Design review of the part built by this model. Coordinates are the model's own, in mm. Face numbers are marked on the shaded views. Round coordinates to 2 decimals unless told otherwise and drop trailing zeros. Order: outer loops, then holes, each group sorted by start corner. A loop starts at its lowest first (then second) coordinate and runs counter-clockwise, first axis right, second up.
from build123d import *

# Parameters (mm, degrees)
SKETCH_1_W          = 420
SKETCH_1_H          = 60
EXTRUDE_1_DEPTH     = 8
SKETCH_2_R          = 30
EXTRUDE_2_DEPTH     = 8
SKETCH_3_W          = 420
SKETCH_3_H          = 8
EXTRUDE_3_DEPTH     = 8
SKETCH_4_R          = 10
CUT_EXTRUDE_1_DEPTH = 481
SKETCH_5_R          = 8
CUT_EXTRUDE_2_DEPTH = 481
CUT_EXTRUDE_3_DEPTH = 455.264240283


with BuildPart() as part:
    # 草图1 → 凸台-拉伸1 (new body)
    with BuildSketch(Plane.XY):
        with Locations((210, 30)):
            Rectangle(SKETCH_1_W, SKETCH_1_H)
    extrude(amount=EXTRUDE_1_DEPTH)

    # 草图2 → 凸台-拉伸2 (add)
    with BuildSketch(Plane.XY):
        with Locations((0, 30)):
            Circle(SKETCH_2_R)
        with Locations((420, 30)):
            Circle(SKETCH_2_R)
    extrude(amount=EXTRUDE_2_DEPTH)

    # 草图3 → 凸台-拉伸3 (add)
    with BuildSketch(Plane.XY.offset(8)):
        with Locations((210, 4)):
            Rectangle(SKETCH_3_W, SKETCH_3_H)
        with Locations((210, 56)):
            Rectangle(SKETCH_3_W, SKETCH_3_H)
    extrude(amount=EXTRUDE_3_DEPTH)

    # 草图4 → 切除-拉伸1 (cut, symmetric)
    with BuildSketch(Plane.XY.offset(8)):
        with Locations((0, 30)):
            Circle(SKETCH_4_R)
    extrude(amount=CUT_EXTRUDE_1_DEPTH, both=True, mode=Mode.SUBTRACT)

    # 草图5 → 切除-拉伸2 (cut, symmetric)
    with BuildSketch(Plane.XY.offset(8)):
        with Locations((420, 30)):
            Circle(SKETCH_5_R)
    extrude(amount=CUT_EXTRUDE_2_DEPTH, both=True, mode=Mode.SUBTRACT)

    # 草图6 → 切除-拉伸3 (cut, through all)
    with BuildSketch(Plane.XY):
        with BuildLine():
            Line((28, 10), (72, 10))
            ThreePointArc((72, 10), (75.577708764, 12.211145618), (75.2, 16.4))
            Line((75.2, 16.4), (53.2, 45.733333333))
            ThreePointArc((53.2, 45.733333333), (50, 47.333333333), (46.8, 45.733333333))
            Line((46.8, 45.733333333), (24.8, 16.4))
            ThreePointArc((24.8, 16.4), (24.422291236, 12.211145618), (28, 10))
        make_face()
        with BuildLine():
            Line((108, 10), (152, 10))
            ThreePointArc((152, 10), (155.577708764, 12.211145618), (155.2, 16.4))
            Line((155.2, 16.4), (133.2, 45.733333333))
            ThreePointArc((133.2, 45.733333333), (130, 47.333333333), (126.8, 45.733333333))
            Line((126.8, 45.733333333), (104.8, 16.4))
            ThreePointArc((104.8, 16.4), (104.422291236, 12.211145618), (108, 10))
        make_face()
        with BuildLine():
            Line((188, 10), (232, 10))
            ThreePointArc((232, 10), (235.577708764, 12.211145618), (235.2, 16.4))
            Line((235.2, 16.4), (213.2, 45.733333333))
            ThreePointArc((213.2, 45.733333333), (210, 47.333333333), (206.8, 45.733333333))
            Line((206.8, 45.733333333), (184.8, 16.4))
            ThreePointArc((184.8, 16.4), (184.422291236, 12.211145618), (188, 10))
        make_face()
        with BuildLine():
            Line((268, 10), (312, 10))
            ThreePointArc((312, 10), (315.577708764, 12.211145618), (315.2, 16.4))
            Line((315.2, 16.4), (293.2, 45.733333333))
            ThreePointArc((293.2, 45.733333333), (290, 47.333333333), (286.8, 45.733333333))
            Line((286.8, 45.733333333), (264.8, 16.4))
            ThreePointArc((264.8, 16.4), (264.422291236, 12.211145618), (268, 10))
        make_face()
        with BuildLine():
            Line((348, 10), (392, 10))
            ThreePointArc((392, 10), (395.577708764, 12.211145618), (395.2, 16.4))
            Line((395.2, 16.4), (373.2, 45.733333333))
            ThreePointArc((373.2, 45.733333333), (370, 47.333333333), (366.8, 45.733333333))
            Line((366.8, 45.733333333), (344.8, 16.4))
            ThreePointArc((344.8, 16.4), (344.422291236, 12.211145618), (348, 10))
        make_face()
        with BuildLine():
            Line((68, 50), (112, 50))
            ThreePointArc((112, 50), (115.577708764, 47.788854382), (115.2, 43.6))
            Line((115.2, 43.6), (93.2, 14.266666667))
            ThreePointArc((93.2, 14.266666667), (90, 12.666666667), (86.8, 14.266666667))
            Line((86.8, 14.266666667), (64.8, 43.6))
            ThreePointArc((64.8, 43.6), (64.422291236, 47.788854382), (68, 50))
        make_face()
        with BuildLine():
            Line((148, 50), (192, 50))
            ThreePointArc((192, 50), (195.577708764, 47.788854382), (195.2, 43.6))
            Line((195.2, 43.6), (173.2, 14.266666667))
            ThreePointArc((173.2, 14.266666667), (170, 12.666666667), (166.8, 14.266666667))
            Line((166.8, 14.266666667), (144.8, 43.6))
            ThreePointArc((144.8, 43.6), (144.422291236, 47.788854382), (148, 50))
        make_face()
        with BuildLine():
            Line((228, 50), (272, 50))
            ThreePointArc((272, 50), (275.577708764, 47.788854382), (275.2, 43.6))
            Line((275.2, 43.6), (253.2, 14.266666667))
            ThreePointArc((253.2, 14.266666667), (250, 12.666666667), (246.8, 14.266666667))
            Line((246.8, 14.266666667), (224.8, 43.6))
            ThreePointArc((224.8, 43.6), (224.422291236, 47.788854382), (228, 50))
        make_face()
        with BuildLine():
            Line((308, 50), (352, 50))
            ThreePointArc((352, 50), (355.577708764, 47.788854382), (355.2, 43.6))
            Line((355.2, 43.6), (333.2, 14.266666667))
            ThreePointArc((333.2, 14.266666667), (330, 12.666666667), (326.8, 14.266666667))
            Line((326.8, 14.266666667), (304.8, 43.6))
            ThreePointArc((304.8, 43.6), (304.422291236, 47.788854382), (308, 50))
        make_face()
    extrude(amount=CUT_EXTRUDE_3_DEPTH, mode=Mode.SUBTRACT)


solid = part.part
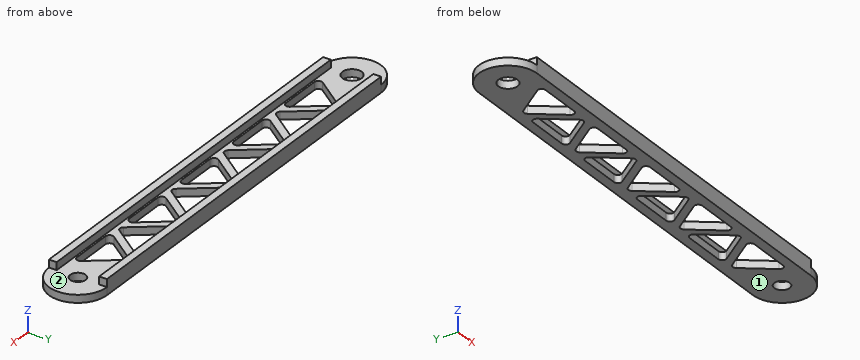
1) Take a section at A-A on x = 321.5. Give the boundary of the cut face in (y, z).
Results:
outline: (0, 0) - (21.33, 0) - (21.33, 8) - (8, 8) - (8, 16) - (0, 16) - close; (50, 0) - (60, 0) - (60, 16) - (52, 16) - (52, 8) - (50, 8) - close
2) The part is to be moulded in two halves that separate along Y. For the marked faces 1 and 2, say which applies: released by +Y, released by -Y, zero draft, split by the parting line, or undercut.
Results:
face 1: zero draft
face 2: undercut
3) Clearance check with flat-ended pins moving along their axes: P1, Ø2.5, axis at x = 254, z = 6, coming from the -Y side; P2, Ø6.5, axis at y = 4.5, z = 13, coming from the +X side; P3, Ø8, axis at y = 21, z = 14, coming from the +X side; P4, Ø4, axis at y = 55.5, z = 12.5, coming from the -X side. State where each tip first meets the part, or that it passes through.
Results:
P1: stops at y = 0
P2: stops at x = 420
P3: passes through
P4: stops at x = 0
4) Take a section at D-D on x = 400. Give the boundary of the cut face in (y, z).
Results:
outline: (0, 0) - (60, 0) - (60, 16) - (52, 16) - (52, 8) - (8, 8) - (8, 16) - (0, 16) - close
5) Take a section at B-B on y = 30. State how many separate pieces and enclosed holes the cut face has, plus the area to 3 significant figures.
Results:
separate pieces: 12
enclosed holes: 0
area: 1,390 mm2
6) To check wall thickness, follow line 1 along Y through (x, z) = (0, 4.5); line 2 along X through (y, z) = (10.5, 4.5); line 3 along Y through (x, z) = (420, 4.25). State the ranges of each line that lie inside material, in increasing order.
Results:
line 1: y = 0 to 20, 40 to 60
line 2: x = -22.8 to 26.06, 73.94 to 106.06, 153.94 to 186.06, 233.94 to 266.06, 313.94 to 346.06, 393.94 to 442.8
line 3: y = 0 to 22, 38 to 60
